from build123d import *

# Parameters (mm, degrees)
SKETCH_1_W               = 73
SKETCH_1_H               = 52
SKETCH_1_W_2             = 67
SKETCH_1_H_2             = 46
EXTRUDE_1_DEPTH          = 30
SKETCH_1_2_W             = 67
SKETCH_1_2_H             = 46
EXTRUDE_2_DEPTH          = 3
CUT_EXTRUDE_1_DEPTH      = 69.067980725
CUT_EXTRUDE_1_DEPTH_BACK = 69.067980725
SKETCH_2_W               = 62.268542554
SKETCH_2_H               = 8.657438287
SKETCH_3_W               = 5
SKETCH_3_H               = 5
SKETCH_3_R               = 1.5
EXTRUDE_3_DEPTH          = 5
CUT_EXTRUDE_2_DEPTH      = 85.858706094
CUT_EXTRUDE_2_DEPTH_BACK = 85.858706094
SKETCH_4_W               = 39.317133882
SKETCH_4_H               = 8.764149171
CUT_EXTRUDE_3_DEPTH      = 88.521425948
CUT_EXTRUDE_3_DEPTH_BACK = 88.521425948
SKETCH_5_W               = 25.853493498
SKETCH_5_H               = 9.668476694
SKETCH_6_R               = 2.613718533
CUT_EXTRUDE_4_DEPTH      = 56.921820428


with BuildPart() as part:
    # Sketch 1 → Extrude 1 (new body)
    with BuildSketch(Plane(origin=(0, 0, 0), x_dir=(1, 0, 0), z_dir=(0, 1, 0))):
        Rectangle(SKETCH_1_W, SKETCH_1_H)
        Rectangle(SKETCH_1_W_2, SKETCH_1_H_2, mode=Mode.SUBTRACT)
    extrude(amount=EXTRUDE_1_DEPTH)

    # Sketch 1_2 → Extrude 2 (add)
    with BuildSketch(Plane(origin=(0, 0, 0), x_dir=(1, 0, 0), z_dir=(0, 1, 0))):
        Rectangle(SKETCH_1_2_W, SKETCH_1_2_H)
    extrude(amount=EXTRUDE_2_DEPTH)

    # Sketch 2 → Cut-Extrude 1 (cut, two sides: drawn at the far end of the back side and taken through both)
    with BuildSketch(Plane.XY.offset(-23).offset(-CUT_EXTRUDE_1_DEPTH_BACK)):
        with Locations((0, 9.350523915)):
            Rectangle(SKETCH_2_W, SKETCH_2_H)
    extrude(amount=CUT_EXTRUDE_1_DEPTH + CUT_EXTRUDE_1_DEPTH_BACK, mode=Mode.SUBTRACT)

    # Sketch 3 → Extrude 3 (add)
    # profile 1 of 4: a face of its own
    with BuildSketch(Plane(origin=(0, 0, 0), x_dir=(1, 0, 0), z_dir=(0, 1, 0))):
        with Locations((39, 23.5)):
            Rectangle(SKETCH_3_W, SKETCH_3_H)
        with Locations(Location((39, 23.5, 0), (0, 0, 270))):
            Circle(SKETCH_3_R, mode=Mode.SUBTRACT)
    # profile 2 of 4: a face of its own
    with BuildSketch(Plane(origin=(0, 0, 0), x_dir=(1, 0, 0), z_dir=(0, 1, 0))):
        with Locations((39, -23.5)):
            Rectangle(SKETCH_3_W, SKETCH_3_H)
        with Locations(Location((39, -23.5, 0), (0, 0, 90))):
            Circle(SKETCH_3_R, mode=Mode.SUBTRACT)
    # profile 3 of 4: a face of its own
    with BuildSketch(Plane(origin=(0, 0, 0), x_dir=(1, 0, 0), z_dir=(0, 1, 0))):
        with Locations((-39, -23.5)):
            Rectangle(SKETCH_3_W, SKETCH_3_H)
        with Locations(Location((-39, -23.5, 0), (0, 0, 270))):
            Circle(SKETCH_3_R, mode=Mode.SUBTRACT)
    # profile 4 of 4: a face of its own
    with BuildSketch(Plane(origin=(0, 0, 0), x_dir=(1, 0, 0), z_dir=(0, 1, 0))):
        with Locations((-39, 23.5)):
            Rectangle(SKETCH_3_W, SKETCH_3_H)
        with Locations(Location((-39, 23.5, 0), (0, 0, 90))):
            Circle(SKETCH_3_R, mode=Mode.SUBTRACT)
    extrude(amount=EXTRUDE_3_DEPTH)

    # Sketch 4 → Cut-Extrude 2 (cut, two sides: drawn at the far end of the back side and taken through both)
    with BuildSketch(Plane.ZY.offset(-33.5).offset(-CUT_EXTRUDE_2_DEPTH_BACK)):
        with Locations((0, 8.573599651)):
            Rectangle(SKETCH_4_W, SKETCH_4_H)
    extrude(amount=CUT_EXTRUDE_2_DEPTH + CUT_EXTRUDE_2_DEPTH_BACK, mode=Mode.SUBTRACT)

    # Sketch 5 → Cut-Extrude 3 (cut, two sides: drawn at the far end of the back side and taken through both)
    with BuildSketch(Plane(origin=(36.5, 0, 0), x_dir=(0, 0, -1), z_dir=(1, 0, 0)).offset(-CUT_EXTRUDE_3_DEPTH_BACK)):
        with Locations((0, 25.165761653)):
            Rectangle(SKETCH_5_W, SKETCH_5_H)
    extrude(amount=CUT_EXTRUDE_3_DEPTH + CUT_EXTRUDE_3_DEPTH_BACK, mode=Mode.SUBTRACT)

    # Sketch 6 → Cut-Extrude 4 (cut, through all)
    with BuildSketch(Plane(origin=(0, 3, 0), x_dir=(1, 0, 0), z_dir=(0, 1, 0))):
        with Locations(Location((-29.37891044, 5.538923259, 0), (0, 0, 270))):
            Circle(SKETCH_6_R)
    extrude(amount=-CUT_EXTRUDE_4_DEPTH, mode=Mode.SUBTRACT)


solid = part.part
CAD build for the part. Positions are in the model's coordinates, mm. A direction names the side the tool comes from. Coordinates: 2 decimals unless noted, no trailing zeros. Loops run counter-clockwise (first coordinate to the right, second up) from the corner with the lowest first, then second, coordinate; pieces in that order, holes last. Notation, with made-up numbers: (49.5, 79) -> (69.5, 79) arc R25 cw to (69.5, 92) -> close; hole circle Ø1 at (9, 6.5). An arc over 180 degrees is marked (long way). One line per item, written item: value.
1. Slice it at C-C on x = -39. Write the cut outline in (y, z), and give its area (3 significant figures).
Answers:
outline: (0, -26) -> (5, -26) -> (5, -25) -> (0, -25) -> close; (0, -22) -> (5, -22) -> (5, -21) -> (0, -21) -> close; (0, 21) -> (5, 21) -> (5, 22) -> (0, 22) -> close; (0, 25) -> (5, 25) -> (5, 26) -> (0, 26) -> close
area: 20.0 mm^2
2. Slice it at A-A on x = 23. Write the cut outline in (y, z).
Answers:
outline: (0, -26) -> (5.02, -26) -> (5.02, -23) -> (3, -23) -> (3, 23) -> (5.02, 23) -> (5.02, 26) -> (0, 26) -> close; (13.68, -26) -> (30, -26) -> (30, -23) -> (13.68, -23) -> close; (13.68, 23) -> (30, 23) -> (30, 26) -> (13.68, 26) -> close
3. Slice it at D-D on z = -9. Write the cut outline in (x, y).
Answers:
outline: (-36.5, 0) -> (36.5, 0) -> (36.5, 4.19) -> (33.5, 4.19) -> (33.5, 3) -> (-33.5, 3) -> (-33.5, 4.19) -> (-36.5, 4.19) -> close; (-36.5, 12.96) -> (-33.5, 12.96) -> (-33.5, 20.33) -> (-36.5, 20.33) -> close; (33.5, 12.96) -> (36.5, 12.96) -> (36.5, 20.33) -> (33.5, 20.33) -> close
4. Which spindle directions (+Z, -Z, +X, -X, +Y, -Y) get a long thin tool onto all of the face, cutting with end or side? Do faces 4 (the face through (-40, 5, -25)), 5 (the face through (0, 13.679, 24)), 6 (the face through (0, 3, 0)), 7 (the face through (38, 5, -25)). Say none if no direction does.
Answers:
face 4: +Z, -Z, -X, +Y
face 5: +Z, -Z
face 6: +Y
face 7: +Z, -Z, +X, +Y
5. Drill centre lines: line 1 (X direction, y = 2.2, z = 23.5); line 2 (Y direction, x = -34.5, z = -15.5); line 3 (Z direction, x = 6, y = 14). Where is each one in solid material? Low to high. Write a range as [from, to].
Answers:
line 1: x = [-41.5, -40.5], [-37.5, 37.5], [40.5, 41.5]
line 2: y = [0, 4.19], [12.96, 30]
line 3: z = [-26, -23], [23, 26]
6. Slice it at B-B on y = 24.5. Write the cut outline in (x, z).
Answers:
outline: (-36.5, -26) -> (36.5, -26) -> (36.5, -12.93) -> (33.5, -12.93) -> (33.5, -23) -> (-33.5, -23) -> (-33.5, -12.93) -> (-36.5, -12.93) -> close; (-36.5, 12.93) -> (-33.5, 12.93) -> (-33.5, 23) -> (33.5, 23) -> (33.5, 12.93) -> (36.5, 12.93) -> (36.5, 26) -> (-36.5, 26) -> close
7. Pull direction Z, two halves, no side cores. Call faces 1 (the face through (39, 2, -21)), 2 (the face through (-31.134, 9, -25)), 3 (the face through (-1, 15, 26)): pulls with the +Z half, pulls with the -Z half, needs draft (parallel to the pull), parting line crosses it, or undercut.
Answers:
face 1: undercut
face 2: needs draft
face 3: pulls with the +Z half
8. Flat gauge pins, fed straight in: P1, Ø3.5, axis at y = 8, z = -24, coming from the -X side; P2, Ø3, axis at x = -29.38, z = -5.54, coming from the +Y side; P3, Ø1.5, axis at x = 39.5, z = 22.5, coming from the +Y side; P4, Ø6, axis at x = 5, z = -7, coming from the +Y side. Where does each tip first touch, or does it go through?
Answers:
P1: stops at x = -36.5
P2: passes through
P3: stops at y = 5
P4: stops at y = 3
